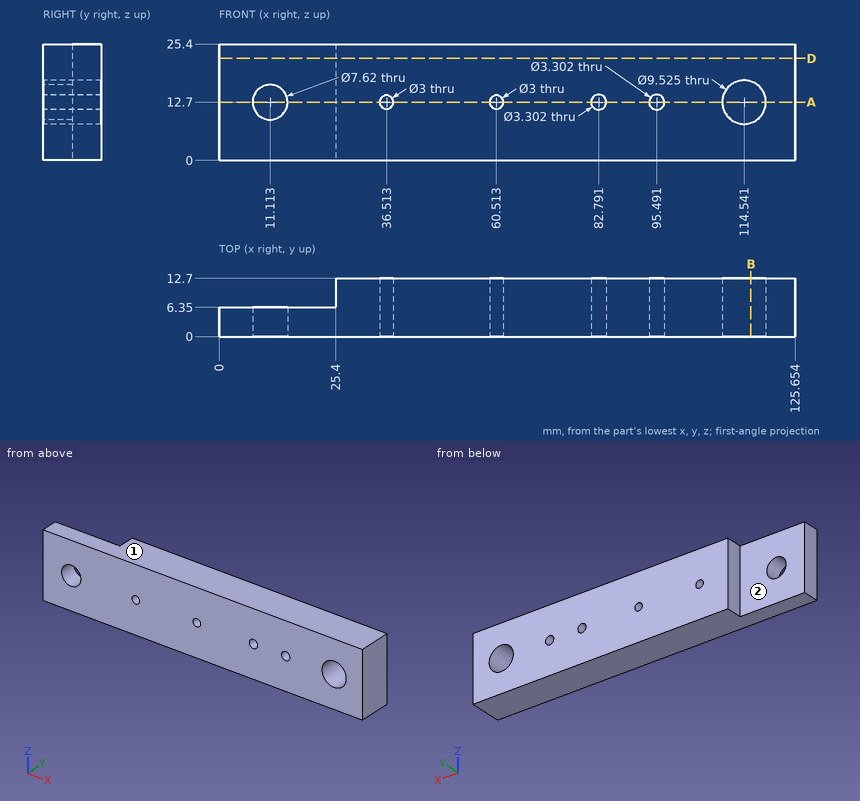
Print and shaded views of the part. All mm, measured from the part's lowest x, y and z. A direction names the side the tool comes from. Give positions to 0.01 mm unless a question says otherwise; leave off trailing zeros. Order: outer loops, then holes, each group sorted by start corner. A loop starts at its lowest first (then second) coordinate and runs counter-clockwise, first axis right, second up. Notation, with made-up numbers: (76.5, 61.5) - (84.5, 61.5) arc R18 ccw to (84.5, 92.5) - close; hole circle Ø8 at (-38, 25). An arc over 180 degrees is marked (long way). Use a Markdown table: item, result.
1) 3-axis set-ups, long thin cutter, end or side, ignore diameter. For the marked faces 1 and 2: which of +Z, -Z, +X, -X, +Y, -Y reach the whole face in a straight line?
Checked values:
| item | result |
|---|---|
| face 1 | +Z, +X, -X, +Y, -Y |
| face 2 | +Z, -Z, -X, +Y |
2) Saw through at B-B on x = 116. List the corners of the cut face in (y, z).
Checked values:
| item | result |
|---|---|
| outline | (0, 0) - (12.7, 0) - (12.7, 8.17) - (0, 8.17) - close; (0, 17.23) - (12.7, 17.23) - (12.7, 25.4) - (0, 25.4) - close |
3) Saw through at D-D on z = 22.25. List the corners of the cut face in (x, y).
Checked values:
| item | result |
|---|---|
| outline | (0, 0) - (125.65, 0) - (125.65, 12.7) - (25.4, 12.7) - (25.4, 6.35) - (0, 6.35) - close |
4) Saw through at A-A on z = 12.7. Count the separate pieces of the cut face and the enclosed holes in it, plus the area to 4 significant figures.
Checked values:
| item | result |
|---|---|
| separate pieces | 7 |
| enclosed holes | 0 |
| area | 1,105 mm² |
5) Probe L1, parallel to X at y = 7.75, z = 12.7; L2, parallel to Z at x = 114.5, y = 4; L3, parallel to X at y = 12, z = 13.75 (1 decimal). List the from-to ranges inside material, lowest first. Write a range as from..to.
Checked values:
| item | result |
|---|---|
| L1 | 25.4..35.01, 38.01..59.01, 62.01..81.14, 84.44..93.84, 97.14..109.78, 119.3..125.65 |
| L2 | 0..7.94, 17.46..25.4 |
| L3 | 25.4..35.4, 37.6..59.4, 61.6..81.5, 84.1..94.2, 96.8..109.9, 119.2..125.7 |
6) Flat gauge pins, fed straight in: P1, Ø8.5, axis at x = 114.54, z = 12.7, coming from the -Y side; P2, Ø5, axis at x = 14, z = 6.5, coming from the +Y side; P3, Ø1.9, axis at y = 10, z = 9, coming from the -X side. Where does each tip first touch, or does it go through?
Checked values:
| item | result |
|---|---|
| P1 | through |
| P2 | y = 6.35 |
| P3 | x = 25.4 |
